Part model, mm, in its own coordinate system. A direction names the side the tool comes from. Coordinates: 2 decimals unless noted, no trailing zeros. Loops run counter-clockwise (first coordinate to the right, second up) from the corner with the lowest first, then second, coordinate; pieces in that order, holes last. Notation, with made-up numbers: M 33,28.5 L 77,28.5 A27 ccw 77,56.5 Z; hole C 64.5,85 d1. An arc over 180 degrees is marked long. Use a Markdown table: item, result. Add a question column.
1) Band-saw the part on A-A (z = 0.5). List the corners of the cut face in (x, y), plus the area to 3 significant figures.
2) Band-saw the part on C-C (x = -0.5). List the corners of the cut face in (y, z).
3) Band-saw the part on D-D (y = 2.75). List the corners of the cut face in (x, z).
4) Tool access for faces 4 (the flat face through (-3, 1, -2.25)), 5 (the cylindrical face through (0, 2, -3)), 6 (the flat face through (3, 1, -2.25)): list every direction of +Z, -Z, +X, -X, +Y, -Y with a clear straight run to the whole face (end or side of a thin tool).
5) Pin check, flat tips, straight feed: pin 1 Ø2 at (y, z) = (4, 6.5) entering from -X; pin 2 Ø2 at (x, z) = (-0.5, 5.5) entering from +Y (3 decimals); pin 3 Ø2 at (x, z) = (1.5, 0.5) entering from +Y; pin 4 Ø2 at (x, z) = (3, -1) entering from -Y. Stop position of each tip, or through.
6) Wall check: probe 1 along X at (y, z) = (7.5, -0.25); probe 2 along Z at (x, y) = (0.75, 10); probe 3 along Z at (x, y) = (-3.25, 2.5). Give the ranges that are in metal, low to high. Write a range as from..to.
7) Band-saw the part on B-B (y = 9.5). List the corners of the cut face in (x, z), plus the area to 3 significant figures.
8) Pull direction X, two halves, no side cores. Call faces 1 (the cylindrical face through (0.26, 1.19, 6.22)), 2 (the flat face through (0, 3, 8.25)), 3 (the flat face through (0, 6, 2.35)): released by +X, released by -X, zero draft, split by the parting line, or undercut.
from build123d import *

# Parameters (mm, degrees)
CROQUIS1_W              = 8.3
CROQUIS1_H              = 8.5
CROQUIS1_W_2            = 4.5
CROQUIS1_H_2            = 4.7
SALIENTE_EXTRUIR1_DEPTH = 12
CORTAR_EXTRUIR3_START   = -8.5
CORTAR_EXTRUIR3_DEPTH   = 8.5
CROQUIS3_R              = 2
SALIENTE_EXTRUIR2_DEPTH = 4
CORTAR_EXTRUIR4_START   = -2
CORTAR_EXTRUIR4_DEPTH   = 2


# Read off the part's stored shape, not the designer's step: Cortar-Extruir3
with BuildPart() as part:
    # Croquis1 → Saliente-Extruir1 (new body)
    with BuildSketch(Plane(origin=(0, 0, 0), x_dir=(1, 0, 0), z_dir=(0, 1, 0))):
        Rectangle(CROQUIS1_W, CROQUIS1_H)
        Rectangle(CROQUIS1_W_2, CROQUIS1_H_2, mode=Mode.SUBTRACT)
    extrude(amount=SALIENTE_EXTRUIR1_DEPTH)

    # Cortar-Extruir3 outline → Cortar-Extruir3 (cut)
    with BuildSketch(Plane(origin=(0, 0, -4.25), x_dir=(-1, 0, 0), z_dir=(0, 0, -1)).offset(CORTAR_EXTRUIR3_START)):
        with BuildLine():
            Line((0, 0), (4.15, 0))
            Line((4.15, 0), (4.15, 0.499191196))
            ThreePointArc((4.15, 0.499191196), (2.089957646, 0.125245986), (0, 0))
        make_face()
        with BuildLine():
            Line((-4.15, 0.499191196), (-4.15, 0))
            Line((-4.15, 0), (0, 0))
            ThreePointArc((0, 0), (-2.089957646, 0.125245986), (-4.15, 0.499191196))
        make_face()
    extrude(amount=CORTAR_EXTRUIR3_DEPTH, mode=Mode.SUBTRACT)

    # Croquis3 → Saliente-Extruir2 (add)
    with BuildSketch(Plane.XY.offset(4.25)):
        with Locations(Location((0, 3.175, 0), (0, 0, 180))):
            Circle(CROQUIS3_R)
    extrude(amount=SALIENTE_EXTRUIR2_DEPTH)

    # Croquis4 → Cortar-Extruir4 (cut)
    with BuildSketch(Plane(origin=(0, 0, -4.25), x_dir=(-1, 0, 0), z_dir=(0, 0, -1)).offset(CORTAR_EXTRUIR4_START)):
        with BuildLine():
            Line((-4.15, 2.565894737), (-4.15, 0.499191196))
            ThreePointArc((-4.15, 0.499191196), (0, 0), (4.15, 0.499191196))
            Line((4.15, 0.499191196), (4.15, 2.565894737))
            ThreePointArc((4.15, 2.565894737), (0, 2), (-4.15, 2.565894737))
        make_face()
    extrude(amount=CORTAR_EXTRUIR4_DEPTH, mode=Mode.SUBTRACT)


solid = part.part
Entries:
| question | item | result |
|---|---|---|
| 1 | outline | M -4.15,0.5 A17.5 ccw -2.25,0.15 L -2.25,12 L -4.15,12 Z; M 2.25,0.15 A17.5 ccw 4.15,0.5 L 4.15,12 L 2.25,12 Z |
| 1 | area | 44.4 mm2 |
| 2 | outline | M 0.01,2.35 L 12,2.35 L 12,4.25 L 5.11,4.25 L 5.11,8.25 L 1.24,8.25 L 1.24,4.25 L 0.01,4.25 Z; M 2.01,-4.25 L 12,-4.25 L 12,-2.35 L 2.01,-2.35 Z |
| 3 | outline | M -4.15,-4.25 L 4.15,-4.25 L 4.15,4.25 L 1.95,4.25 L 1.95,8.25 L -1.95,8.25 L -1.95,4.25 L -4.15,4.25 Z; hole M -2.25,-2.35 L 2.25,-2.35 L 2.25,2.35 L -2.25,2.35 Z |
| 4 | face 4 | -Z, -X, -Y |
| 4 | face 5 | -Z, -Y |
| 4 | face 6 | -Z, +X, -Y |
| 5 | pin 1 | x = -2 |
| 5 | pin 2 | y = 5.175 |
| 5 | pin 3 | y = 12 |
| 5 | pin 4 | y = 0.15 |
| 6 | probe 1 | -4.15..-2.25, 2.25..4.15 |
| 6 | probe 2 | -4.25..-2.35, 2.35..4.25 |
| 6 | probe 3 | -4.25..4.25 |
| 7 | outline | M -4.15,-4.25 L 4.15,-4.25 L 4.15,4.25 L -4.15,4.25 Z; hole M -2.25,-2.35 L 2.25,-2.35 L 2.25,2.35 L -2.25,2.35 Z |
| 7 | area | 49.4 mm2 |
| 8 | face 1 | split by the parting line |
| 8 | face 2 | zero draft |
| 8 | face 3 | undercut |
